Can you work these out from the drawing? Everything is in mm from the part's minimum corner. A direction names the side the tool comes from. Give positions to 0.01 mm unless a question says otherwise; leave off trailing zeros. Write each loop counter-clockwise with the first axis right and the second up, starting at its lowest first coordinate (ties: lowest second). Pieces come first, ordered by that corner, then holes. Notation, with made-up numbers: (69, 34) - (122, 34) arc R16 ccw to (122, 42) - close; hole circle Ø5 at (70, 69.5). An arc over 180 degrees is marked (long way). Use a Markdown table: item, result.
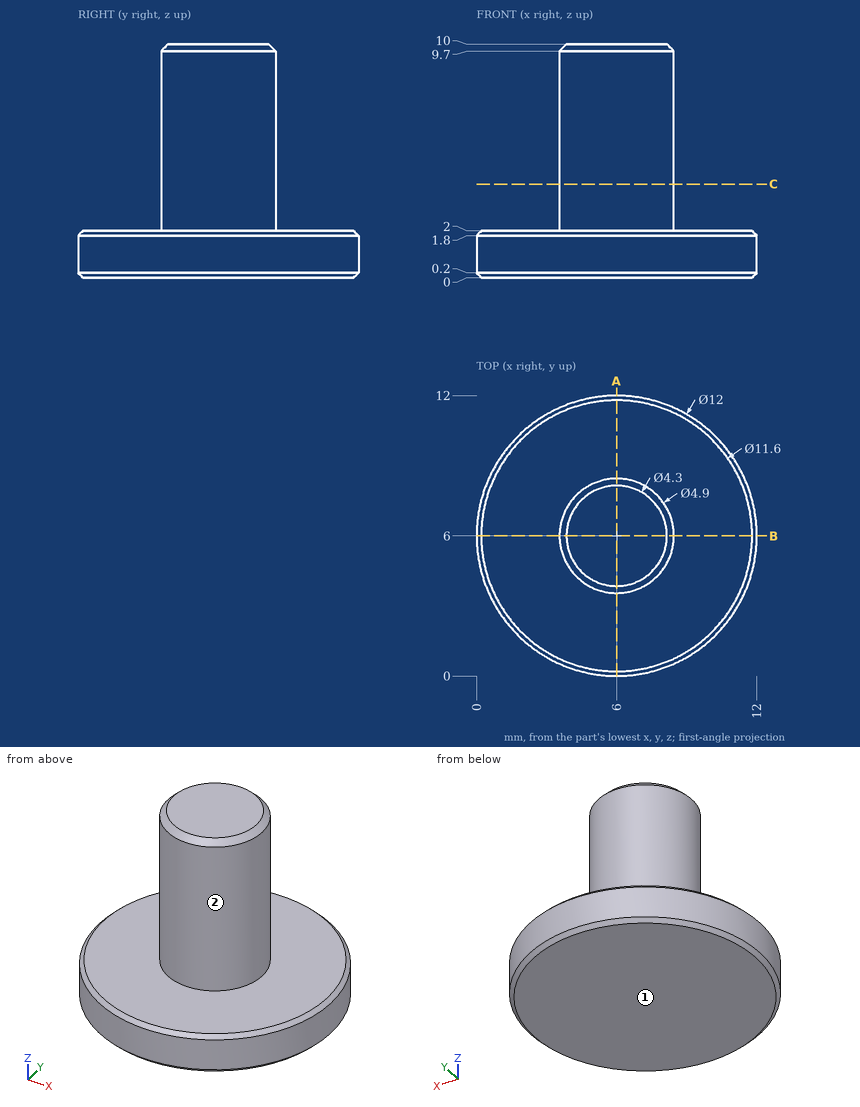
Item 1: Will these pins go through, and if not, where does the flat tip stop? pin 1 Ø6 at (x, z) = (6.5, 7) entering from -Y; pin 2 Ø6 at (x, y) = (5, 5) entering from -Z; pin 3 Ø2 at (y, z) = (7.5, 8.5) entering from -X; pin 4 Ø1 at (y, z) = (4.5, 2) entering from -X.
Values:
| item | result |
|---|---|
| pin 1 | stops at y = 3.55 |
| pin 2 | stops at z = 0 |
| pin 3 | stops at x = 3.6 |
| pin 4 | stops at x = 0.09 |
Item 2: For the marked faces 1 and 2, which set-ups out of +Z, -Z, +X, -X, +Y, -Y let a thin tool reach every point of the face, with its end or its side?
Values:
| item | result |
|---|---|
| face 1 | -Z, +X, -X, +Y, -Y |
| face 2 | +Z |
Item 3: If we section it at A-A, the plane x = 6: Write out the boundary of the cut face in (y, z), plus the area to 3 significant figures.
Values:
| item | result |
|---|---|
| outline | (0, 0.2) - (0.2, 0) - (11.8, 0) - (12, 0.2) - (12, 1.8) - (11.8, 2) - (8.45, 2) - (8.45, 9.7) - (8.15, 10) - (3.85, 10) - (3.55, 9.7) - (3.55, 2) - (0.2, 2) - (0, 1.8) - close |
| area | 63.0 mm2 |
Item 4: If we section it at C-C, the plane z = 4: Write out the boundary of the cut face in (x, y), plus the area to 3 significant figures.
Values:
| item | result |
|---|---|
| outline | circle Ø4.9 at (6, 6) |
| area | 18.9 mm2 |
Item 5: I need wall thicknesses on line 1 along Z through (x, y) = (3, 10); line 2 along X through (y, z) = (7.25, 1.5); line 3 along Y through (x, z) = (0.75, 1). Which ranges of each line are inside material? Lowest first, please. Write a range as [from, to].
Values:
| item | result |
|---|---|
| line 1 | z = [0, 2] |
| line 2 | x = [0.13, 11.87] |
| line 3 | y = [3.1, 8.9] |
